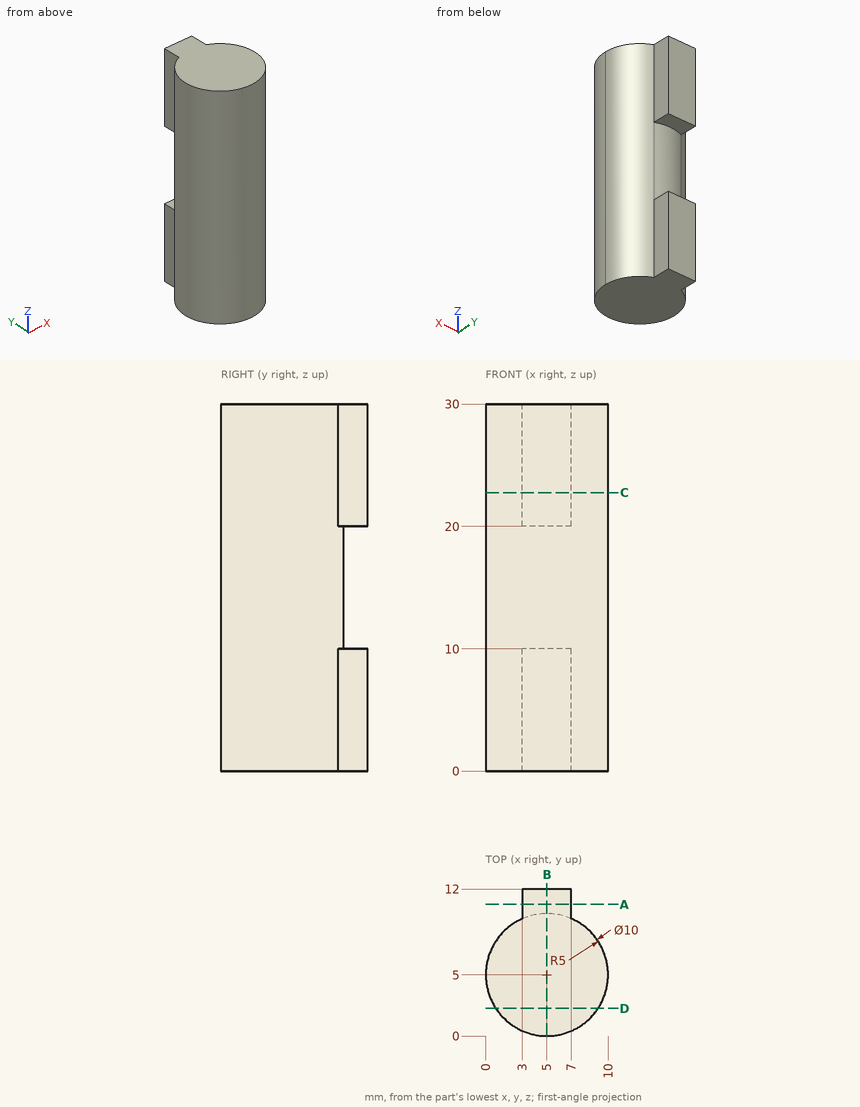
Source: three-view drawing plus pictorial views. Frame: mm from the lowest corner of the part. Coordinates: 2 decimals unless noted, no trailing zeros. Write each loop counter-clockwise with the first axis right and the second up, starting at its lowest first coordinate (ties: lowest second). Pieces come first, ordered by that corner, then holes. Notation, with made-up numbers: (16.5, 63.5) - (22.5, 63.5) arc R25 cw to (22.5, 75.5) - close; hole circle Ø9 at (5, 77.5). An arc over 180 degrees is marked (long way). Return JSON: item names as keys, results as strings.
Item 1: Section query C-C (z = 22.75). Output: boundary loops of the cut face in (x, y).
Completed:
{"outline": "(3, 9.58) arc R5 ccw (long way) to (7, 9.58) - (7, 12) - (3, 12) - close"}
Item 2: Section query B-B (x = 5). Output: boundary loops of the cut face in (y, z), and give its area (3 significant figures).
Completed:
{"outline": "(0, 0) - (12, 0) - (12, 10) - (10, 10) - (10, 20) - (12, 20) - (12, 30) - (0, 30) - close", "area": "340 mm2"}
Item 3: Section query D-D (y = 2.25). Output: boundary loops of the cut face in (x, z).
Completed:
{"outline": "(0.82, 0) - (9.18, 0) - (9.18, 30) - (0.82, 30) - close"}
Item 4: Pin query (flat end, axial travel): pin 1 Ø1.9 at (y, z) = (11.5, 23.5) entering from -X; pin 2 Ø2.5 at (y, z) = (10, 6) entering from -X; pin 3 Ø1.5 at (y, z) = (9, 8.5) entering from +X. Return the tip coordinate at first contact, or that it passes through.
Completed:
{"pin 1": "stops at x = 3", "pin 2": "stops at x = 1.69", "pin 3": "stops at x = 8.8"}
Item 5: Section query A-A (y = 10.75). Output: boundary loops of the cut face in (x, z), and give its area (3 significant figures).
Completed:
{"outline": "(3, 0) - (7, 0) - (7, 10) - (3, 10) - close; (3, 20) - (7, 20) - (7, 30) - (3, 30) - close", "area": "80.0 mm2"}
Item 6: Line query: L1, parallel to X at y = 11.5, z = 22; L2, parallel to Z at x = 3.25, y = 10.75; L3, parallel to Y at x = 4.75, z = 12.75. Output: solid intervals per line, ascending.
Completed:
{"L1": "x = 3 to 7", "L2": "z = 0 to 10, 20 to 30", "L3": "y = 0.01 to 9.99"}
